Read the model definition and answer for the solid it produces. Units are mm, in the model's axes. Face numbers are marked on the shaded views. A direction names the side the tool comes from. Coordinates: 2 decimals unless noted, no trailing zeros. Loops run counter-clockwise (first coordinate to the right, second up) from the corner with the lowest first, then second, coordinate; pieces in that order, holes last. Notation, with made-up numbers: M -9,71.5 L 7,71.5 A29 ccw 7,95.5 Z; hole C 68.5,30 d7. An arc over 180 degrees is marked long. Use one line per item in the form item = value. Start each with the question number.
1. For a pull along Z with two mould halves and no side action, classify the marked faces 1, 2 and 3 as released by +Z, released by -Z, zero draft, split by the parting line, or undercut.
2. Flat-ended cylindrical pins translate along their axes: pin 1 (1.9 mm diameter, centred on x = 9.51, z = 6.35, fed in from -Y); pin 2 (4.5 mm diameter, centred on x = 0, z = 4.5, fed in from +Y). Find the tip coordinate at first contact, or state that the pin passes through.
3. The part is cut by section B-B (y = 0). Give the vertices of the cut face in (x, z), plus the area to 3 significant figures.
4. The part is cut by section A-A (z = 6.35). Give the number of separate pieces and of enclosed holes in the cut face, plus the area to 3 significant figures.
5. The part is cut by section D-D (x = -3). Give the vertices of the cut face in (y, z), plus the area to 3 significant figures.
6. A tool of negligible diameter and unlimited length cuts with its end or side. For the marked faces 4 and 5, from which of +Z, -Z, +X, -X, +Y, -Y can it reach the whole face along a straight path? Write none if from no direction.
7. Find the intervals of material crossed by probe 1 along X at (y, z) = (7.25, 6.25); probe 2 along Z at (x, y) = (3.75, -12); probe 3 along Z at (x, y) = (0, -13.6), in increasing order. Write a range as [from, to].
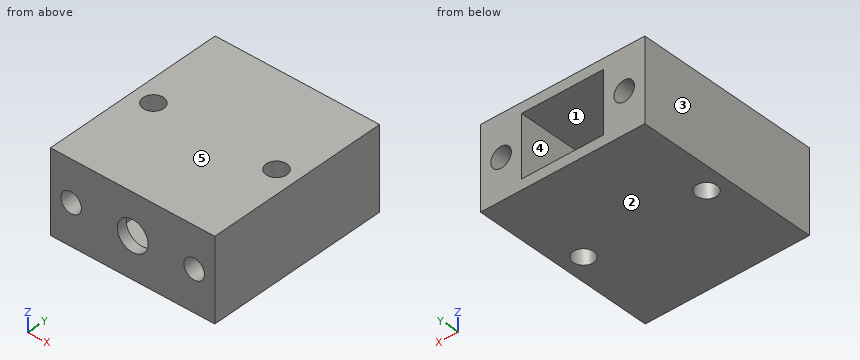
from build123d import *

# Parameters (mm, degrees)
F0_W     = 25.4
F0_H     = 28.575
F0_R     = 1.5875
F1_DEPTH = 12.7
F2_W     = 12.7
F2_H     = 9.4996
F3_DEPTH = 27.0002
F4_R     = 2.38125
F5_DEPTH = 1.5758
F6_R     = 1.5875
F7_DEPTH = 11.43
F8_R     = 1.5875
F9_DEPTH = 11.43


with BuildPart() as f1:
    # F0 (on Top) → F1 (new body)
    with BuildSketch(Plane.XY):
        Rectangle(F0_W, F0_H)
        with Locations((-9.5123, 0)):
            Circle(F0_R, mode=Mode.SUBTRACT)
        with Locations((9.5123, 0)):
            Circle(F0_R, mode=Mode.SUBTRACT)
    extrude(amount=F1_DEPTH)

    # F2 (on face) → F3 (cut)
    with BuildSketch(Plane(origin=(0, 14.2875, 0), x_dir=(-1, 0, 0), z_dir=(0, 1, 0))):
        with Locations((0, 6.35)):
            Rectangle(F2_W, F2_H)
    extrude(amount=-F3_DEPTH, mode=Mode.SUBTRACT)

    # F4 (on face) → F5 (cut, through all)
    with BuildSketch(Plane(origin=(0, -12.7127, 0), x_dir=(-1, 0, 0), z_dir=(0, 1, 0))):
        with Locations((0, 6.35)):
            Circle(F4_R)
    extrude(amount=-F5_DEPTH, mode=Mode.SUBTRACT)

    # F6 (on face) → F7 (cut)
    with BuildSketch(Plane.XZ.offset(14.2875)):
        with Locations((-9.5123, 6.35)):
            Circle(F6_R)
        with Locations((9.5123, 6.35)):
            Circle(F6_R)
    extrude(amount=-F7_DEPTH, mode=Mode.SUBTRACT)

    # F8 (on face) → F9 (cut)
    with BuildSketch(Plane(origin=(0, 14.2875, 0), x_dir=(-1, 0, 0), z_dir=(0, 1, 0))):
        with Locations((-9.5123, 6.35)):
            Circle(F8_R)
        with Locations((9.5123, 6.35)):
            Circle(F8_R)
    extrude(amount=-F9_DEPTH, mode=Mode.SUBTRACT)


solid = f1.part
Computed values:
q1.face_1 = undercut
q1.face_2 = released by -Z
q1.face_3 = zero draft
q2.pin_1 = -2.86
q2.pin_2 = -12.71
q3.outline = M -12.7,0 L -11.1,0 L -11.1,12.7 L -12.7,12.7 Z; M -7.92,0 L 7.92,0 L 7.92,12.7 L -7.92,12.7 Z; M 11.1,0 L 12.7,0 L 12.7,12.7 L 11.1,12.7 Z; hole M -6.35,1.6 L 6.35,1.6 L 6.35,11.1 L -6.35,11.1 Z
q3.area = 121 mm²
q4.separate_pieces = 2
q4.enclosed_holes = 2
q4.area = 214 mm²
q5.outline = M -14.29,0 L 14.29,0 L 14.29,1.6 L -12.71,1.6 L -12.71,11.1 L 14.29,11.1 L 14.29,12.7 L -14.29,12.7 Z
q5.area = 106 mm²
q6.face_4 = +Y
q6.face_5 = +Z, +X, -X, +Y, -Y
q7.probe_1 = [-12.7, -11.1], [-7.93, -6.35], [6.35, 7.93], [11.1, 12.7]
q7.probe_2 = [0, 1.6], [11.1, 12.7]
q7.probe_3 = [0, 3.97], [8.73, 12.7]
